Design review of the part shown in the three views and the two pictorial views. Dimensions are in mm from the part's minimum x, y and z. A direction names the side the tool comes from. Give positions to 0.01 mm unless a question says otherwise; leave off trailing zeros. Order: outer loops, then holes, each group sorted by start corner. A loop starts at its lowest first (then second) coordinate and runs counter-clockwise, first axis right, second up. Notation, with made-up numbers: M 8,13.25 L 66,13.25 A21 ccw 66,28.25 Z; hole C 74,59 d6. An arc over 180 degrees is marked long. Answer as a JSON object with one key per item and string values.
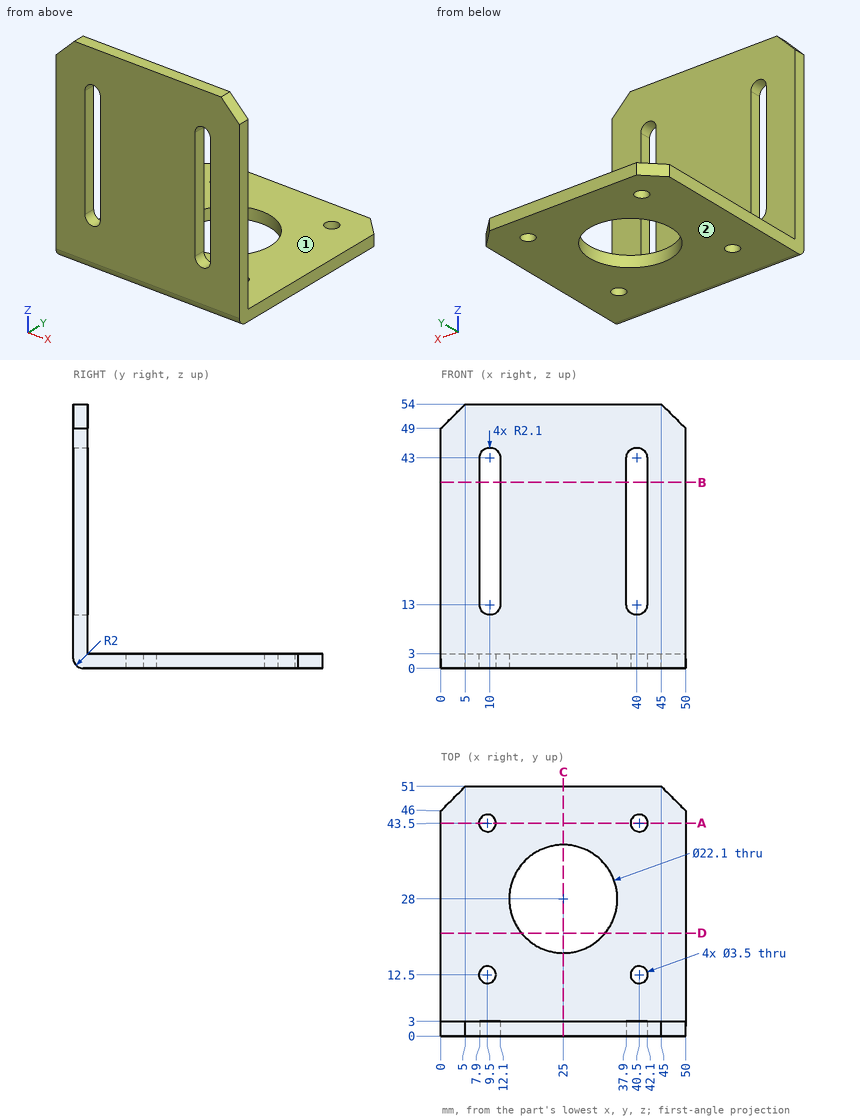
(1) Insertion check: pin 1 (24 mm diameter, centred on x = 31, y = 32, fed in from +Z); pin 2 (25 mm diameter, centred on x = 33, z = 38, fed in from +Y); pin 3 (13.5 mm diameter, centred on x = 25, y = 28, fed in from +Z). Each pin has a flat end and moves straight along its axis. Give the tip position at first contact, or say it passes through.
Checked values:
{"pin 1": "stops at z = 3", "pin 2": "stops at y = 3", "pin 3": "passes through"}
(2) We need section B-B (z = 38). Write out the cut boundary in (x, y).
Checked values:
{"outline": "M 0,0 L 7.9,0 L 7.9,3 L 0,3 Z; M 12.1,0 L 37.9,0 L 37.9,3 L 12.1,3 Z; M 42.1,0 L 50,0 L 50,3 L 42.1,3 Z"}
(3) We need section A-A (y = 43.5). Write out the cut boundary in (x, z).
Checked values:
{"outline": "M 0,0 L 7.75,0 L 7.75,3 L 0,3 Z; M 11.25,0 L 38.75,0 L 38.75,3 L 11.25,3 Z; M 42.25,0 L 50,0 L 50,3 L 42.25,3 Z"}
(4) Tool access review of the marked faces 1 and 2: name each direction out of +Z, -Z, +X, -X, +Y, -Y from which nothing blocks a thin tool from reaching the whole face with its end or side.
Checked values:
{"face 1": "+Z, +X, -X, +Y", "face 2": "-Z, +X, -X, +Y, -Y"}
(5) To check wall thickness, follow L1, parallel to Y at x = 40, z = 2; L2, parallel to Y at x = 40.5, z = 0.7; L3, parallel to Y at x = 43, z = 17. State the ranges of each line that lie inside material, in increasing order. Write a range as from..to.
Checked values:
{"L1": "y = 0..10.82, 14.18..41.82, 45.18..51", "L2": "y = 0.48..10.75, 14.25..41.75, 45.25..51", "L3": "y = 0..3"}
(6) We need section D-D (y = 21). Write out the cut boundary in (x, z).
Checked values:
{"outline": "M 0,0 L 16.45,0 L 16.45,3 L 0,3 Z; M 33.55,0 L 50,0 L 50,3 L 33.55,3 Z"}
(7) We need section C-C (x = 25). Write out the cut boundary in (y, z).
Checked values:
{"outline": "M 0,2 A2 ccw 2,0 L 16.95,0 L 16.95,3 L 3,3 L 3,54 L 0,54 Z; M 39.05,0 L 51,0 L 51,3 L 39.05,3 Z"}
